Design review of the part built by this model. Coordinates are the model's own, in mm. Face numbers are marked on the shaded views. A direction names the side the tool comes from. Coordinates: 2 decimals unless noted, no trailing zeros. Write each loop counter-clockwise with the first axis right and the second up, starting at its lowest first coordinate (ties: lowest second). Pieces come first, ordered by that corner, then holes. Notation, with made-up numbers: (88.25, -31.75) -> (136.25, -31.75) arc R11 ccw to (136.25, -14.75) -> close; hole circle Ø10 at (58, 40). An arc over 180 degrees is marked (long way). One line per question, with ' | ' between items. Start each with the question number.
Q1. For the marked faces 3, 4, 5, 6 and 7, list the 3-axis set-ups (+Z, -Z, +X, -X, +Y, -Y) from which the entire face can be reached by the end or side of a thin tool; tool diameter is ignored.
Q2. For P1, Ø3, axis at y = 3, z = 36.5, coming from the -X side; P2, Ø4, axis at x = -2, z = -29, coming from the -Y side; P3, Ø4, axis at x = -42, y = 2, coming from the +Z side; P4, Ø3.5, axis at x = 23.75, z = -41.14, coming from the -Y side, all flat-tipped, find the tip position at first contact; note any pin that passes through.
Q3. Add section C-C on z = 11.5. State the section outline as (x, y) points, and give its area (3 significant figures).
Q4. Add section D-D on y = 3.75. Give the number of separate pieces and of enclosed holes in the cut face, and give its area (3 significant figures).
Q5. Add section B-B on x = 0. State the section outline as (y, z) points.
Q6. Wall thickness on probe 1 along Z at (x, y) = (-47.5, 1.25); probe 2 along Z at (x, y) = (5, -1.25); probe 3 along Z at (x, y) = (21, -0.5): over which ranges is each line inside the solid? List them lowest first.
Q7. Draft analysis for pull direction X (two halves, no side actions). For the marked faces 1 and 2, state which applies: pulls with the +X half, pulls with the -X half, needs draft (parallel to the pull), parting line crosses it, or undercut.
Q8. Add section A-A on z = 0. State the section outline as (x, y) points, and give its area (3 significant figures).
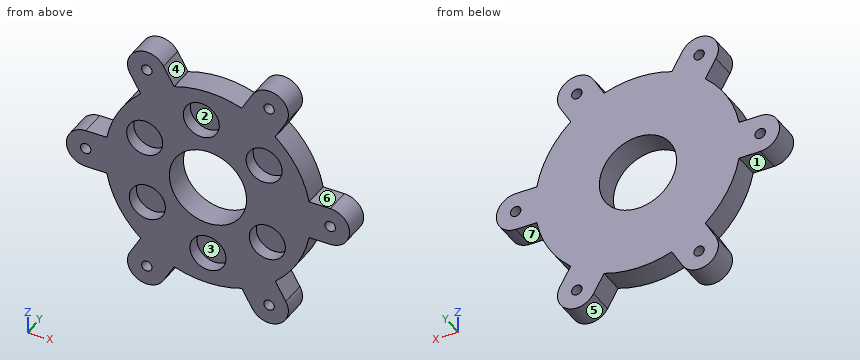
from build123d import *

# Parameters (mm, degrees)
SKETCH1_R                  = 25
SKETCH1_R_2                = 15
BOSS_EXTRUDE1_DEPTH        = 5
SKETCH6_R                  = 40
SKETCH6_R_2                = 25
BOSS_EXTRUDE3_DEPTH        = 10
SKETCH7_R                  = 7
CUT_EXTRUDE1_DEPTH         = 5
BOSS_EXTRUDE4_DEPTH        = 10
TAP_DRILL_FOR_10_32_TAP1_D = 4.0386
CIRPATTERN1_COUNT          = 6


with BuildPart() as part:
    # Sketch1 → Boss-Extrude1 (new, symmetric)
    with BuildSketch(Plane(origin=(0, 0, 0), x_dir=(1, 0, 0), z_dir=(0, 1, 0))):
        with Locations(Location((0, 0, 0), (0, 0, 270))):
            Circle(SKETCH1_R)
        with Locations(Location((0, 0, 0), (0, 0, 270))):
            Circle(SKETCH1_R_2, mode=Mode.SUBTRACT)
    extrude(amount=BOSS_EXTRUDE1_DEPTH, both=True)

    # Sketch6 → Boss-Extrude3 (add)
    with BuildSketch(Plane(origin=(0, 5, 0), x_dir=(1, 0, 0), z_dir=(0, 1, 0))):
        with Locations(Location((0, 0, 0), (0, 0, 270))):
            Circle(SKETCH6_R)
        Circle(SKETCH6_R_2, mode=Mode.SUBTRACT)
    extrude(amount=-BOSS_EXTRUDE3_DEPTH)

    # Sketch7 → Cut-Extrude1 (cut)
    with BuildSketch(Plane.XZ.offset(5)):
        with Locations(Location((21.817216858, 16.740939298, 0), (0, 0, 270))):
            Circle(SKETCH7_R)
        with Locations(Location((-2.585088545, 27.378227065, 0), (0, 0, 270))):
            Circle(SKETCH7_R)
        with Locations(Location((-24.565103939, 12.361458995, 0), (0, 0, 270))):
            Circle(SKETCH7_R)
        with Locations(Location((-23.52702738, -14.238292828, 0), (0, 0, 270))):
            Circle(SKETCH7_R)
        with Locations(Location((0, -27.5, 0), (0, 0, 270))):
            Circle(SKETCH7_R)
        with Locations(Location((23.055532132, -14.989744431, 0), (0, 0, 270))):
            Circle(SKETCH7_R)
    extrude(amount=-CUT_EXTRUDE1_DEPTH, mode=Mode.SUBTRACT)

    # Sketch8 → Boss-Extrude4 (add)
    with BuildSketch(Plane(origin=(0, 5, 0), x_dir=(1, 0, 0), z_dir=(0, 1, 0))):
        with BuildLine():
            Line((47.5, 7.5), (39.290584114, 7.5))
            Line((39.290584114, 7.5), (39.290584114, -7.5))
            Line((39.290584114, -7.5), (47.5, -7.5))
            ThreePointArc((47.5, -7.5), (55, 0), (47.5, 7.5))
        make_face()
    boss_extrude4 = extrude(amount=-BOSS_EXTRUDE4_DEPTH)

    # Tap Drill for #10-32 Tap1 (through all)
    with Locations(Plane(origin=(0, 5, 0), x_dir=(1, 0, 0), z_dir=(0, 1, 0))):
        with Locations((47.5, 0)):
            tap_drill_for_10_32_tap1 = Hole(TAP_DRILL_FOR_10_32_TAP1_D / 2)

    # CirPattern1: Boss-Extrude4, Tap Drill for #10-32 Tap1 ×6 about axis
    cirpattern1_axis = Axis((0, 0, 0), (0, 1, 0))
    add([boss_extrude4.rotate(cirpattern1_axis, i * 360 / CIRPATTERN1_COUNT) for i in range(1, CIRPATTERN1_COUNT)])
    add([tap_drill_for_10_32_tap1.rotate(cirpattern1_axis, i * 360 / CIRPATTERN1_COUNT) for i in range(1, CIRPATTERN1_COUNT)], mode=Mode.SUBTRACT)


solid = part.part
Output values:
1) face 3: -Y | face 4: +Z, +Y, -Y | face 5: +Y, -Y | face 6: +Z, +X, +Y, -Y | face 7: -Z, +X, +Y, -Y
2) P1: stops at x = -30.56 | P2: stops at y = 0 | P3: stops at z = 7.5 | P4: passes through
3) outline: (-38.31, -5) -> (-31.51, -5) -> (-31.51, 0) -> (-17.62, 0) -> (-17.62, -5) -> (-9.63, -5) -> (-9.63, 5) -> (-38.31, 5) -> close; (9.63, -5) -> (17.18, -5) -> (17.18, 0) -> (26.46, 0) -> (26.46, -5) -> (38.31, -5) -> (38.31, 5) -> (9.63, 5) -> close | area: 458 mm2
4) separate pieces: 1 | enclosed holes: 7 | area: 5,470 mm2
5) outline: (-5, -40) -> (5, -40) -> (5, -15) -> (-5, -15) -> (-5, -20.5) -> (0, -20.5) -> (0, -34.5) -> (-5, -34.5) -> close; (-5, 15) -> (5, 15) -> (5, 40) -> (-5, 40) -> (-5, 33.88) -> (0, 33.88) -> (0, 20.87) -> (-5, 20.87) -> close
6) probe 1: z = -7.5 to -2.02, 2.02 to 7.5 | probe 2: z = -39.69 to -32.4, -22.6 to -14.14, 14.14 to 39.69 | probe 3: z = -48.11 to -21.68, -8.3 to 9.79, 23.69 to 48.11
7) face 1: needs draft | face 2: undercut
8) outline: (-55, -5) -> (-49.52, -5) -> (-49.52, 5) -> (-55, 5) -> close; (-45.48, -5) -> (-15, -5) -> (-15, 5) -> (-45.48, 5) -> close; (15, -5) -> (45.48, -5) -> (45.48, 5) -> (15, 5) -> close; (49.52, -5) -> (55, -5) -> (55, 5) -> (49.52, 5) -> close | area: 719 mm2
